Source: CAD feature listing. Evaluate the final solid. Frame: model axes, mm. A direction names the side the tool comes from. Coordinates: 2 decimals unless noted, no trailing zeros. Write each loop counter-clockwise with the first axis right and the second up, starting at its lowest first coordinate (ties: lowest second). Pieces come first, ordered by that corner, then holes. Notation, with made-up numbers: (74, -6.5) -> (79, -6.5) arc R19 cw to (79, 3.5) -> close; hole circle Ø6 at (7, 31). An arc over 180 degrees is marked (long way). Write item = value, one per line.
from build123d import *

# Parameters (mm, degrees)
SKETCH_1_W               = 330
SKETCH_1_H               = 80
EXTRUDE_1_DEPTH          = 5
SKETCH_2_R               = 5
CUT_EXTRUDE_1_DEPTH      = 5
SKETCH_3_R               = 4
CUT_EXTRUDE_2_DEPTH      = 10
SKETCH_4_W               = 88
SKETCH_4_H               = 20
EXTRUDE_2_DEPTH          = 10
SKETCH_5_R               = 15
CUT_EXTRUDE_3_DEPTH      = 10
SKETCH_6_R               = 8
EXTRUDE_3_DEPTH          = 15
F_6_0MM_1_D              = 6
CUT_EXTRUDE_4_DEPTH      = 7
HOLE_WIZARD_M4_1_D       = 3.3
FILLET_1_R               = 10
SKETCH_13_R              = 6.969385005
EXTRUDE_5_DEPTH          = 5
SKETCH_14_W              = 5
SKETCH_14_H              = 75
EXTRUDE_6_DEPTH          = 80
SKETCH_15_W              = 20
SKETCH_15_H              = 5
EXTRUDE_7_DEPTH          = 80
EXTRUDE_8_DEPTH          = 5
SKETCH_17_R              = 3
CUT_EXTRUDE_5_DEPTH      = 5
FILLET_2_R               = 1
FILLET_3_R               = 1
CUT_EXTRUDE_6_DEPTH      = 100
F_3_0MM_1_D              = 3
F_3_0MM_1_DEPTH          = 7.5
F_3_0MM_1_TIP            = 0.901290929
SKETCH_21_R              = 2.5
CUT_EXTRUDE_7_DEPTH      = 10
PATTERN_CIRCULAR_1_COUNT = 4
CUT_EXTRUDE_START        = -5
SKETCH_25_R              = 5.25
CUT_EXTRUDE_8_DEPTH      = 86


with BuildPart() as part:
    # 草图1 → 凸台-拉伸1 (new body)
    with BuildSketch(Plane.XY):
        Rectangle(SKETCH_1_W, SKETCH_1_H)
    extrude(amount=EXTRUDE_1_DEPTH)

    # 草图2 → 切除-拉伸1 (cut)
    with BuildSketch(Plane.XY.offset(5)):
        with Locations((-145, 0)):
            Circle(SKETCH_2_R)
    extrude(amount=-CUT_EXTRUDE_1_DEPTH, mode=Mode.SUBTRACT)

    # 草图3 → 切除-拉伸2 (cut)
    with BuildSketch(Plane.XY.offset(5)):
        with Locations((-45, 0)):
            Circle(SKETCH_3_R)
    extrude(amount=-CUT_EXTRUDE_2_DEPTH, mode=Mode.SUBTRACT)

    # 草图4 → 凸台-拉伸2 (add)
    with BuildSketch(Plane.XY.offset(5)):
        with Locations((-47, 0)):
            Rectangle(SKETCH_4_W, SKETCH_4_H)
    extrude(amount=EXTRUDE_2_DEPTH)

    # 草图5 → 切除-拉伸3 (cut)
    with BuildSketch(Plane.XY.offset(5)):
        with Locations((32.5, 0)):
            Circle(SKETCH_5_R)
    extrude(amount=-CUT_EXTRUDE_3_DEPTH, mode=Mode.SUBTRACT)

    # 草图6 → 凸台-拉伸3 (add)
    with BuildSketch(Plane(origin=(0, 0, 0), x_dir=(-1, 0, 0), z_dir=(0, 0, -1))):
        with Locations((145, 0)):
            Circle(SKETCH_6_R)
    extrude(amount=-EXTRUDE_3_DEPTH)

    # Ø6.0mm 暗销孔1 (through all)
    with Locations(Plane.XY.offset(15)):
        with Locations((-145, 0)):
            Hole(F_6_0MM_1_D / 2)

    # 草图10 → 切除-拉伸4 (cut)
    with BuildSketch(Plane.XY.offset(15)):
        with BuildLine():
            Line((-91, 5.1), (-3, 5.1))
            ThreePointArc((-3, 5.1), (2.1, 0), (-3, -5.1))
            Line((-3, -5.1), (-91, -5.1))
            ThreePointArc((-91, -5.1), (-96.1, 0), (-91, 5.1))
        make_face()
    extrude(amount=-CUT_EXTRUDE_4_DEPTH, mode=Mode.SUBTRACT)

    # M4 螺纹孔1 (through all)
    with Locations(Plane(origin=(0, 0, 0), x_dir=(-1, 0, 0), z_dir=(0, 0, -1))):
        with Locations((-2.25, -26.5), (-2.25, -1.5), (-62.75, -26.5), (-62.75, -1.5)):
            Hole(HOLE_WIZARD_M4_1_D / 2)

    # 圆角1
    fillet_1_edges = [part.edges().sort_by_distance(p)[0] for p in [
        (-165, 40, 2.5),
        (-165, -40, 2.5),
    ]]
    fillet(fillet_1_edges, radius=FILLET_1_R)

    # 草图13 → 凸台-拉伸5 (add)
    with BuildSketch(Plane.XY.offset(5)):
        with Locations((-45, 0)):
            Circle(SKETCH_13_R)
    extrude(amount=-EXTRUDE_5_DEPTH)

    # 草图14 → 凸台-拉伸6 (add)
    with BuildSketch(Plane.XZ.offset(40)):
        with Locations((162.5, -37.5)):
            Rectangle(SKETCH_14_W, SKETCH_14_H)
    extrude(amount=-EXTRUDE_6_DEPTH)

    # 草图15 → 凸台-拉伸7 (add)
    with BuildSketch(Plane.XZ.offset(40)):
        with Locations((150, -72.5)):
            Rectangle(SKETCH_15_W, SKETCH_15_H)
    extrude(amount=-EXTRUDE_7_DEPTH)

    # 草图16 → 凸台-拉伸8 (add)
    with BuildSketch(Plane.XZ.offset(40)):
        Polygon((5, 5), (5, 0), (140, -55), (140, -75), (165, -75), (165, 5), align=None)
    extrude_8 = extrude(amount=-EXTRUDE_8_DEPTH)

    # 镜向1: 凸台-拉伸8 across plane
    add(extrude_8.mirror(Plane.ZX))

    # 草图17 → 切除-拉伸5 (cut)
    with BuildSketch(Plane(origin=(0, 0, -75), x_dir=(-1, 0, 0), z_dir=(0, 0, -1))):
        with Locations((-152, -15)):
            Circle(SKETCH_17_R)
        with Locations((-152, 15)):
            Circle(SKETCH_17_R)
    extrude(amount=-CUT_EXTRUDE_5_DEPTH, mode=Mode.SUBTRACT)

    # 圆角2
    fillet_2_edges = [part.edges().sort_by_distance(p)[0] for p in [
        (-75, -40, 0),
        (5, -40, 5),
        (-165, 0, 0),
        (-162.071067812, 37.071067812, 0),
        (-162.071067812, -37.071067812, 0),
        (-165, 0, 5),
        (-162.071067812, 37.071067812, 5),
        (-162.071067812, -37.071067812, 5),
        (165, 0, -75),
        (165, 0, 5),
        (152.5, -40, -75),
        (152.5, 40, -75),
        (140, -40, -65),
        (140, 40, -65),
        (72.5, -40, -27.5),
        (5, 40, 5),
        (-75, 40, 0),
        (72.5, 40, -27.5),
        (165, 40, -35),
        (165, -40, -35),
    ]]
    fillet(fillet_2_edges, radius=FILLET_2_R)

    # 圆角3
    fillet_3_edges = [part.edges().sort_by_distance(p)[0] for p in [
        (-47, -10, 15),
        (-47, 10, 15),
        (-47, 5.1, 15),
        (-47, -5.1, 15),
    ]]
    fillet(fillet_3_edges, radius=FILLET_3_R)

    # 草图18 → 切除-拉伸6 (cut)
    with BuildSketch(Plane(origin=(-3, 0, 0), x_dir=(0, 0, -1), z_dir=(1, 0, 0))):
        with BuildLine():
            Line((-15, -6.1), (-15, -9))
            ThreePointArc((-15, -9), (-14.707106781, -9.707106781), (-14, -10))
            Line((-14, -10), (-5, -10))
            Line((-5, -10), (-5, 10))
            Line((-5, 10), (-14, 10))
            ThreePointArc((-14, 10), (-14.707106781, 9.707106781), (-15, 9))
            Line((-15, 9), (-15, 6.1))
            ThreePointArc((-15, 6.1), (-14.707106781, 5.392893219), (-14, 5.1))
            Line((-14, 5.1), (-8, 5.1))
            Line((-8, 5.1), (-8, -5.1))
            Line((-8, -5.1), (-14, -5.1))
            ThreePointArc((-14, -5.1), (-14.707106781, -5.392893219), (-15, -6.1))
        make_face()
    extrude(amount=-CUT_EXTRUDE_6_DEPTH, mode=Mode.SUBTRACT)

    # Ø3.0mm 暗销孔1
    with Locations(Plane.XY.offset(5)):
        with Locations((-14.5, -10), (-14.5, 10), (-47, 10), (-47, -10), (-79.5, -10), (-79.5, 10)):
            Hole(F_3_0MM_1_D / 2, depth=F_3_0MM_1_DEPTH)
            with Locations((0, 0, -(F_3_0MM_1_DEPTH + F_3_0MM_1_TIP / 2))):  # 118° drill point
                Cone(0, F_3_0MM_1_D / 2, F_3_0MM_1_TIP, mode=Mode.SUBTRACT)

    # 草图21 → 切除-拉伸7 (cut)
    with BuildSketch(Plane(origin=(165, 0, 0), x_dir=(0, 0, -1), z_dir=(1, 0, 0))):
        with Locations((35, 0)):
            Circle(SKETCH_21_R)
    extrude(amount=-CUT_EXTRUDE_7_DEPTH, mode=Mode.SUBTRACT)

    # 草图24 → Ø5.0mm 暗销孔1 (revolve, cut)
    with BuildSketch(Plane(origin=(165, 28.991378029, -6.008621971), x_dir=(0, 0, -1), z_dir=(0, 1, 0))):
        Polygon((0, 0), (0, 13.902151548), (2.5, 12.4), (2.5, 0), align=None)
    f_5_0mm_1 = revolve(axis=Axis((171.35, 28.991378029, -6.008621971), (-1, 0, 0)), mode=Mode.SUBTRACT)

    # 阵列(圆周)1: Ø5.0mm 暗销孔1 ×4 about axis
    pattern_circular_1_axis = Axis((0, 0, -35), (1, 0, 0))
    for i in range(1, PATTERN_CIRCULAR_1_COUNT):
        add(f_5_0mm_1.rotate(pattern_circular_1_axis, i * 360 / PATTERN_CIRCULAR_1_COUNT), mode=Mode.SUBTRACT)

    # 草图25 → 切除-拉伸8 (cut, through all)
    with BuildSketch(Plane.XY.offset(15).offset(CUT_EXTRUDE_START)):
        with Locations((-145, 0)):
            Circle(SKETCH_25_R)
    extrude(amount=-CUT_EXTRUDE_8_DEPTH, mode=Mode.SUBTRACT)


solid = part.part
1) First-contact query: pin 1 Ø8 at (y, z) = (0, -35) entering from +X; pin 2 Ø12 at (x, y) = (38, 31) entering from -Z; pin 3 Ø1 at (y, z) = (24.5, -42) entering from -X; pin 4 Ø5 at (x, y) = (-47, 10) entering from -Z. Flat tips, straight axial feed; report the tip coordinate or a pass-through.
Answer block:
pin_1 = 165
pin_2 = -15.27
pin_3 = 160
pin_4 = 0
2) Cut plane A-A, the plane x = 152. Output: boundary loops of the cut face in (y, z).
Answer block:
outline = (-40, -74) arc R1 ccw to (-39, -75) -> (-18, -75) -> (-18, -70) -> (-35, -70) -> (-35, 0) -> (35, 0) -> (35, -70) -> (18, -70) -> (18, -75) -> (39, -75) arc R1 ccw to (40, -74) -> (40, 4) arc R1 ccw to (39, 5) -> (-39, 5) arc R1 ccw to (-40, 4) -> close; (-12, -75) -> (12, -75) -> (12, -70) -> (-12, -70) -> close
3) Cut plane B-B, the plane x = -20. Output: boundary loops of the cut face in (y, z).
Answer block:
outline = (-40, 1) arc R1 ccw to (-39, 0) -> (39, 0) arc R1 ccw to (40, 1) -> (40, 4) arc R1 ccw to (39, 5) -> (-39, 5) arc R1 ccw to (-40, 4) -> close
4) Material intervals for probe 1 along Y at (x, z) = (-47, 1.35); probe 2 along Y at (x, z) = (2, 1); probe 3 along Y at (x, z) = (143.5, -64.5), sorted ascending. Write a range as [from, to].
Answer block:
probe_1 = [-40, -11.5], [-8.5, 8.5], [11.5, 40]
probe_2 = [-40, -28.13], [-24.87, -3.13], [0.13, 40]
probe_3 = [-40, -35], [35, 40]
5) Pull-direction query (X, two-part tool) for faces 4 (the flat face through (152, -1, -75)), 5 (the cylindrical face through (149.23, -16.15, -72.54)), 6 (the flat face through (160, 0, -43)); classes: +X half, -X half, draft (parallel to the pull), parting line (faces both ways), or undercut.
Answer block:
face_4 = draft
face_5 = undercut
face_6 = -X half
6) Reachability of faces 1 (the flat face through (150, 0, -70)), 2 (the cylindrical face through (-152.39, -3.06, 9.93)), 3 (the cylindrical face through (149.23, 13.85, -72.54)) from +Z, -Z, +X, -X, +Y, -Y: full face, straight path, thin tool, end or side. Return the list, or none.
Answer block:
face_1 = -X
face_2 = +Z
face_3 = -Z
